Could you check a few things on this model? Use its own coordinates, in mm. A direction names the side the tool comes from. Give positions to 0.01 mm unless a question says otherwise; leave off trailing zeros. Order: outer loops, then holes, each group sorted by start corner. A loop starts at its lowest first (then second) coordinate and runs counter-clockwise, first axis right, second up. Notation, with made-up numbers: M 67.5,59.25 L 79.5,59.25 A16 cw 79.5,79.25 Z; hole C 72,0.25 d8. An arc over 180 degrees is marked long. Use a Markdown table: item, result. Add a question column.
Item 1: For faces 1 (the face through (-6, 2, -24.219)), 2 (the face through (6.848, 2, 6)), 3 (the face through (-3.134, 2, 26)), 4 (the face through (5.65, 2, -23)), which set-ups out of +Z, -Z, +X, -X, +Y, -Y let a thin tool reach every point of the face, with its end or its side?
Item 2: Suppose I cut it at A-A on x = -5.5. Write out the boundary of the cut face in (y, z) (3 decimals).
Item 3: I'm going to push a flat-ended pin straight in: pin 1 Ø1 at (x, y) = (2.5, 2) entering from -Z. Where does the tip first touch, or does it pass through?
Item 4: Suppose I cut it at C-C on z = 7. Write out the boundary of the cut face in (x, y) (3 decimals).
Item 5: Suppose I cut it at B-B on z = -12. Write out the boundary of the cut face in (x, y) (3 decimals), plus the area to 3 significant figures.
Item 6: If I drill on L1, parallel to X at y = 1.5, z = 6.5; L2, parallel to Z at x = 2.5, y = 1.35; L3, parallel to X at y = 3.05, z = 24, over which ranges is the centre line in solid material (lowest first)? Write a range as from..to.
Item 7: Suppose I cut it at D-D on y = 2.7. Count the separate pieces of the cut face and the enclosed holes in it, plus the area to 3 significant figures.
Item 8: If we mould it in two halves opening along X, with no side actions, what happens to faces 5 (the face through (0.5, 0, 1.3)), 6 (the face through (9.843, 2, 1)), 7 (the face through (0, 2, -11.218)), 8 (the face through (-1.138, 2, -19))? For each: released by +X, released by -X, zero draft, split by the parting line, or undercut.
from build123d import *

# Parameters (mm, degrees)
SKETCH1_W           = 2.994660031
SKETCH1_H           = 8.000362858
SKETCH1_W_2         = 3.294225957
SKETCH1_H_2         = 3.300262419
SKETCH1_W_3         = 6.488474747
SKETCH1_H_3         = 2.999948682
BOSS_EXTRUDE1_DEPTH = 3.175


with BuildPart() as part:
    # Sketch1 → Boss-Extrude1 (new body)
    with BuildSketch(Plane(origin=(0, 0, 0), x_dir=(1, 0, 0), z_dir=(0, 1, 0))):
        Polygon((-3.134063131, -27.4833399), (-9.123310076, -27.4833399), (-9.123310076, 24.218538917), (-3.134063129, 24.218538917), (-3.134063129, 21.21845839), (-1.137605236, 21.21845839), (-1.137605236, 17.218250104), (-2.3854164, 17.218250104), (-2.3854164, 14.718365303), (-1.137605236, 14.718365303), (-1.137605236, 11.218216013), (1.857303385, 11.218216013), (1.857303385, 14.718365303), (3.105051182, 14.718365303), (3.105051182, 17.218250104), (1.857303385, 17.218250104), (1.857303385, 21.21845839), (5.650440312, 21.21845839), (5.650440312, 24.218538917), (9.842944855, 24.218538917), (9.842944855, -27.4833399), (3.853571177, -27.4833399), (3.853571177, -24.483195893), (1.857303382, -24.483195893), (1.857303382, -21.383140191), (3.10505118, -21.383140191), (3.10505118, -18.883001466), (1.857303382, -18.883001466), (1.857303382, -15.082802129), (-1.137605238, -15.082802129), (-1.137605238, -18.883001466), (-2.385416402, -18.883001466), (-2.385416402, -21.383140191), (-1.137605238, -21.383140191), (-1.137605238, -24.483195893), (-3.134063131, -24.483195893), align=None)
        with Locations((-4.490515563, -6.328244045)):
            Rectangle(SKETCH1_W, SKETCH1_H, mode=Mode.SUBTRACT)
        with Locations((5.201303454, -6.328244045)):
            Rectangle(SKETCH1_W_2, SKETCH1_H_2, mode=Mode.SUBTRACT)
        with Locations((0.908846113, 0.517732338)):
            Rectangle(SKETCH1_W_3, SKETCH1_H_3, mode=Mode.SUBTRACT)
    extrude(amount=BOSS_EXTRUDE1_DEPTH)


solid = part.part
Findings below:
| question | item | result |
|---|---|---|
| 1 | face 1 | -Z, +X, -X, +Y, -Y |
| 1 | face 2 | +Y, -Y |
| 1 | face 3 | +Z, +Y, -Y |
| 1 | face 4 | -Z, +Y, -Y |
| 2 | outline | M 0,-24.219 L 3.175,-24.219 L 3.175,2.328 L 0,2.328 Z; M 0,10.328 L 3.175,10.328 L 3.175,27.483 L 0,27.483 Z |
| 3 | pin 1 | stops at z = -21.22 |
| 4 | outline | M -9.123,0 L -5.988,0 L -5.988,3.175 L -9.123,3.175 Z; M -2.993,0 L 3.554,0 L 3.554,3.175 L -2.993,3.175 Z; M 6.848,0 L 9.843,0 L 9.843,3.175 L 6.848,3.175 Z |
| 5 | outline | M -9.123,0 L -1.138,0 L -1.138,3.175 L -9.123,3.175 Z; M 1.857,0 L 9.843,0 L 9.843,3.175 L 1.857,3.175 Z |
| 5 | area | 50.7 mm^2 |
| 6 | L1 | x = -9.12..-5.99, -2.99..3.55, 6.85..9.84 |
| 6 | L2 | z = -21.22..-17.22, -14.72..-2.02, 0.98..18.88, 21.38..24.48 |
| 6 | L3 | x = -9.12..-1.14, 1.86..9.84 |
| 7 | separate pieces | 1 |
| 7 | enclosed holes | 3 |
| 7 | area | 808 mm^2 |
| 8 | face 5 | zero draft |
| 8 | face 6 | released by +X |
| 8 | face 7 | undercut |
| 8 | face 8 | undercut |
